```python
from build123d import *

# Parameters (mm, degrees)
F2_R     = 1.7145
F3_DEPTH = 9.525
F4_R     = 0.3048


with BuildPart() as f1:
    # F0 (on Front) → F1 (revolve)
    with BuildSketch(Plane.XZ):
        with BuildLine():
            Line((0, 12.573), (0, 0))
            Line((0, 0), (13.843, 0))
            Line((13.843, 0), (13.843, 3.175))
            Line((13.843, 3.175), (24.003, 3.175))
            Line((24.003, 3.175), (24.003, 4.7625))
            Line((24.003, 4.7625), (32.591104, 4.7625))
            ThreePointArc((32.591104, 4.7625), (27.96219, 10.43933), (20.955, 12.573))
            Line((20.955, 12.573), (0, 12.573))
        make_face()
    revolve(axis=Axis((6.9215, 0, 0), (-1, 0, 0)))

    # F2 (on face) → F3 (cut)
    with BuildSketch(Plane(origin=(0, 0, 0), x_dir=(0, -1, 0), z_dir=(-1, 0, 0))):
        with Locations((0, 9.525)):
            Circle(F2_R)
        with Locations((-9.525, 0)):
            Circle(F2_R)
        with Locations((0, -9.525)):
            Circle(F2_R)
        with Locations((9.525, 0)):
            Circle(F2_R)
    extrude(amount=-F3_DEPTH, mode=Mode.SUBTRACT)

    # F4
    f4_edges = [f1.edges().sort_by_distance(p)[0] for p in [
        (0, 0, -12.573),
    ]]
    fillet(f4_edges, radius=F4_R)


solid = f1.part
```
Work out the finished part from the listing and answer in its coordinate system (mm). A direction names the side the tool comes from. Give positions to 0.01 mm unless a question says otherwise; leave off trailing zeros. Order: outer loops, then holes, each group sorted by start corner. A loop starts at its lowest first (then second) coordinate and runs counter-clockwise, first axis right, second up. Notation, with made-up numbers: (39, 47) -> (55, 47) arc R14 cw to (55, 62) -> close; hole circle Ø10 at (36, 40.5). An arc over 180 degrees is marked (long way). Answer as CSV lines item,"result". Start each with the question number.
(1) Section A-A, the plane x = 6 is taken. Write down the section's boundary in (y, z) (1 decimal), plus the area to 3 significant figures.
(2) Section B-B, the plane x = 19 is taken. Write down the section's boundary in (y, z) (3 decimals).
(3) For a pull along Z with two mould halves and no side action, classify faces 3 (the flat face through (0, 0, 0)), 4 (the cylindrical face through (10.485, -12.274, -2.726)), 5 (the flat face through (9.525, 0, 10)) as released by +Z, released by -Z, zero draft, split by the parting line, or undercut.
(4) Which of the six approach directions +Z, -Z, +X, -X, +Y, -Y give full straight-line access (tool end or side, diameter ignored) to faces 1 (the flat face through (13.843, 0, 0)), 2 (the cylindrical face through (4.7, 7.89, 0.51))?
(5) Consider line 1 along Z through (x, y) = (2, 1); line 2 along Y through (x, z) = (19, 0) (3 decimals); line 3 along X through (y, z) = (-0.75, 0). Determine where each line is inside the solid, lowest interval first.
(6) Each of these flat-tipped pins is pushed along its axis until it touches: pin 1 Ø2 at (x, z) = (18.5, 7) entering from +Y; pin 2 Ø5 at (x, z) = (29, -5) entering from +Y; pin 3 Ø3 at (x, y) = (28, -5) entering from -Z. Where does it stop, or does it pass through?
Entries:
1,outline,"circle Ø25.1 at (0, 0); hole circle Ø3.4 at (-9.5, 0); hole circle Ø3.4 at (0, -9.5); hole circle Ø3.4 at (0, 9.5); hole circle Ø3.4 at (9.5, 0)"
1,area,"460 mm²"
2,outline,"circle Ø25.146 at (0, 0); hole circle Ø6.35 at (0, 0)"
3,face 3,"zero draft"
3,face 4,"split by the parting line"
3,face 5,"undercut"
4,face 1,"+X"
4,face 2,"-X"
5,line 1,"-12.53 to -10.92, -8.13 to 8.13, 10.92 to 12.53"
5,line 2,"-12.573 to -3.175, 3.175 to 12.573"
5,line 3,"0 to 13.84"
6,pin 1,"y = 11.05"
6,pin 2,"y = 10.46"
6,pin 3,"z = -10.35"
